Geometry check sheet. Reference: the model listing, model coordinates, mm. A direction names the side the tool comes from. Round coordinates to 2 decimals unless told otherwise and drop trailing zeros. Order: outer loops, then holes, each group sorted by start corner. A loop starts at its lowest first (then second) coordinate and runs counter-clockwise, first axis right, second up.
(1) Draft check along Y on faces 1 (the face through (-18.5, 41, 28)), 2 (the face through (-9.1, 35.83, 27.46)), 3 (the face through (-21.5, 38, 29)). Enter one of: pulls with the +Y half, pulls with the -Y half, needs draft (parallel to the pull), parting line crosses it, or undercut.
(2) Gauge pin test, flat ends, axial feed: P1, Ø5, axis at y = 38, z = 53, coming from the +X side; P2, Ø12.5, axis at x = -23, y = 33, coming from the +Z side; P3, Ø2.5, axis at x = -12.5, z = 27.5, coming from the +Y side. Record the tip position at first contact, or that the pin passes through.
(3) Thickness scan on L1, parallel to Z at x = -97.05, y = 42.65; L2, parallel to X at y = 37.5, z = 35; L3, parallel to X at y = 43.4, z = 17.5. Record the ranges inside material, lowest first.
(4) Set-up check for faces 4 (the face through (-94.1, 40, 38)), 5 (the face through (-31, 28.4, 29)), 6 (the face through (-70, 26, 59)), 7 (the face through (-28, 28, 30)): record each of +Z, -Z, +X, -X, +Y, -Y from which the full face is reachable in a straight line by a thin tool's end or side.
(5) Cross-section at B-B on z = 49. Enter the section's corners in (x, y).
(6) Cross-section at C-C on x = -23. Enter the section's corners in (y, z).
(7) Cross-section at D-D on y = 25. Enter the section's corners in (x, z).
(8) Cross-section at A-A on y = 30.9. Enter the section's corners in (x, z), and give its area (3 significant figures).
from build123d import *

# Parameters (mm, degrees)
SKIZZE1_W                            = 100
SKIZZE1_H                            = 50
AUFSATZ_LINEAR_AUSTRAGEN1_DEPTH      = 10
SERVOLOCH_R                          = 5
SCHNITT_LINEAR_AUSTRAGEN2_DEPTH      = 11
BREITE_W                             = 60
BREITE_H                             = 17
AUFSATZ_LINEAR_AUSTRAGEN2_DEPTH      = 65
SERVO_W                              = 12.1
SERVO_H                              = 23.5
SERVO_R                              = 1.9
SERVO_R_2                            = 1
SCHNITT_LINEAR_AUSTRAGEN3_DEPTH      = 60
F_1_2MM_SCHIENE_W                    = 10
F_1_2MM_SCHIENE_H                    = 65
AUFSATZ_LINEAR_AUSTRAGEN3_DEPTH      = 1.2
SERVOTIEFER_LEGEN_W                  = 12.1
SERVOTIEFER_LEGEN_H                  = 5
SCHNITT_LINEAR_AUSTRAGEN4_DEPTH      = 7.5
F_10_2MM_SCHIENE_W                   = 5.9
F_10_2MM_SCHIENE_H                   = 65
AUFSATZ_LINEAR_AUSTRAGEN4_DEPTH      = 10.2
SCHNITT_LINEAR_AUSTRAGEN5_DEPTH      = 11
SKIZZE11_W                           = 40
SKIZZE11_H                           = 50
SKIZZE11_R                           = 2
AUFSATZ_LINEAR_AUSTRAGEN5_DEPTH      = 20
SKIZZE12_W                           = 40
SKIZZE12_H                           = 50
SCHNITT_LINEAR_AUSTRAGEN6_DEPTH      = 25
SCHNITT_LINEAR_AUSTRAGEN8_DEPTH      = 3
SCHNITT_LINEAR_AUSTRAGEN9_DEPTH      = 46
SCHNITT_LINEAR_AUSTRAGEN9_DEPTH_BACK = 30
VERRUNDUNG5_R                        = 2
VERRUNDUNG6_R                        = 2
VERRUNDUNG7_R                        = 2
SKIZZE14_R                           = 1.25
SCHNITT_LINEAR_AUSTRAGEN10_DEPTH     = 5


with BuildPart() as part:
    # Skizze1 → Aufsatz-Linear austragen1 (new body)
    with BuildSketch(Plane.XY):
        with Locations((-50, 25)):
            Rectangle(SKIZZE1_W, SKIZZE1_H)
    extrude(amount=AUFSATZ_LINEAR_AUSTRAGEN1_DEPTH)

    # ServoLoch → Schnitt-Linear austragen2 (cut, through all)
    with BuildSketch(Plane.XY.offset(10)):
        with Locations((-22.5, 25)):
            Circle(SERVOLOCH_R)
    extrude(amount=-SCHNITT_LINEAR_AUSTRAGEN2_DEPTH, mode=Mode.SUBTRACT)

    # Breite → Aufsatz-Linear austragen2 (add)
    with BuildSketch(Plane.XY.offset(10)):
        with Locations((-70, 25)):
            Rectangle(BREITE_W, BREITE_H)
    extrude(amount=AUFSATZ_LINEAR_AUSTRAGEN2_DEPTH)

    # Servo → Schnitt-Linear austragen3 (cut)
    with BuildSketch(Plane(origin=(0, 33.5, 0), x_dir=(1, 0, 0), z_dir=(0, 1, 0))):
        with Locations((-70, -43.25)):
            Rectangle(SERVO_W, SERVO_H)
        with Locations((-70, -37.5)):
            Circle(SERVO_R, mode=Mode.SUBTRACT)
        with Locations((-70, -37.5)):
            Circle(SERVO_R)
        with Locations((-70, -29)):
            Circle(SERVO_R_2)
        with Locations((-70, -57.5)):
            Circle(SERVO_R_2)
    extrude(amount=-SCHNITT_LINEAR_AUSTRAGEN3_DEPTH, mode=Mode.SUBTRACT)

    # 1,2mm Schiene → Aufsatz-Linear austragen3 (add)
    with BuildSketch(Plane(origin=(0, 33.5, 0), x_dir=(1, 0, 0), z_dir=(0, 1, 0))):
        with Locations((-95, -42.5)):
            Rectangle(F_1_2MM_SCHIENE_W, F_1_2MM_SCHIENE_H)
        with Locations((-45, -42.5)):
            Rectangle(F_1_2MM_SCHIENE_W, F_1_2MM_SCHIENE_H)
    extrude(amount=AUFSATZ_LINEAR_AUSTRAGEN3_DEPTH)

    # ServoTiefer legen → Schnitt-Linear austragen4 (cut)
    with BuildSketch(Plane(origin=(0, 33.5, 0), x_dir=(1, 0, 0), z_dir=(0, 1, 0))):
        with Locations((-70, -29)):
            Rectangle(SERVOTIEFER_LEGEN_W, SERVOTIEFER_LEGEN_H)
        with Locations((-70, -57.5)):
            Rectangle(SERVOTIEFER_LEGEN_W, SERVOTIEFER_LEGEN_H)
    extrude(amount=-SCHNITT_LINEAR_AUSTRAGEN4_DEPTH, mode=Mode.SUBTRACT)

    # 10,2mm Schiene → Aufsatz-Linear austragen4 (add)
    with BuildSketch(Plane(origin=(0, 34.7, 0), x_dir=(1, 0, 0), z_dir=(0, 1, 0))):
        with Locations((-97.05, -42.5)):
            Rectangle(F_10_2MM_SCHIENE_W, F_10_2MM_SCHIENE_H)
        with Locations((-42.95, -42.5)):
            Rectangle(F_10_2MM_SCHIENE_W, F_10_2MM_SCHIENE_H)
    extrude(amount=AUFSATZ_LINEAR_AUSTRAGEN4_DEPTH)

    # Skizze10 → Schnitt-Linear austragen5 (cut, through all)
    with BuildSketch(Plane.XY.offset(10)):
        Polygon((-100, 44.9), (-94.1, 44.9), (-94.1, 34.7), (-90, 34.7), (-90, 33.5), (-50, 33.5), (-50, 34.7), (-45.9, 34.7), (-45.9, 44.9), (-40, 44.9), (-40, 52.602302565), (-100, 52.602302565), align=None)
    extrude(amount=-SCHNITT_LINEAR_AUSTRAGEN5_DEPTH, mode=Mode.SUBTRACT)

    # Skizze11 → Aufsatz-Linear austragen5 (add)
    with BuildSketch(Plane.XY.offset(10)):
        with Locations((-20, 25)):
            Rectangle(SKIZZE11_W, SKIZZE11_H)
        with Locations((-24, 30.9)):
            Circle(SKIZZE11_R, mode=Mode.SUBTRACT)
    extrude(amount=AUFSATZ_LINEAR_AUSTRAGEN5_DEPTH)

    # Skizze12 → Schnitt-Linear austragen6 (cut)
    with BuildSketch(Plane(origin=(0, 0, 0), x_dir=(-1, 0, 0), z_dir=(0, 0, -1))):
        with Locations((20, 25)):
            Rectangle(SKIZZE12_W, SKIZZE12_H)
    extrude(amount=-SCHNITT_LINEAR_AUSTRAGEN6_DEPTH, mode=Mode.SUBTRACT)

    # Skizze15 → Schnitt-Linear austragen8 (cut)
    with BuildSketch(Plane.XY.offset(30)):
        with BuildLine():
            Line((-21.5, 40.9), (-21.5, 34.4))
            ThreePointArc((-21.5, 34.4), (-21.207106781, 33.692893219), (-20.5, 33.4))
            Line((-20.5, 33.4), (-14, 33.4))
            ThreePointArc((-14, 33.4), (-11.5, 30.9), (-14, 28.4))
            Line((-14, 28.4), (-20.5, 28.4))
            ThreePointArc((-20.5, 28.4), (-21.207106781, 28.107106781), (-21.5, 27.4))
            Line((-21.5, 27.4), (-21.5, 20.9))
            ThreePointArc((-21.5, 20.9), (-24, 18.4), (-26.5, 20.9))
            Line((-26.5, 20.9), (-26.5, 27.4))
            ThreePointArc((-26.5, 27.4), (-26.792893219, 28.107106781), (-27.5, 28.4))
            Line((-27.5, 28.4), (-34, 28.4))
            ThreePointArc((-34, 28.4), (-36.5, 30.9), (-34, 33.4))
            Line((-34, 33.4), (-27.5, 33.4))
            ThreePointArc((-27.5, 33.4), (-26.792893219, 33.692893219), (-26.5, 34.4))
            Line((-26.5, 34.4), (-26.5, 40.9))
            ThreePointArc((-26.5, 40.9), (-24, 43.4), (-21.5, 40.9))
        make_face()
    extrude(amount=-SCHNITT_LINEAR_AUSTRAGEN8_DEPTH, mode=Mode.SUBTRACT)

    # Skizze18 → Schnitt-Linear austragen9 (cut, two sides)
    with BuildSketch(Plane.XY.offset(30)) as schnitt_linear_austragen9_sk:
        Polygon((0, 0), (-100, 0), (-100, 16.5), (-8.5, 16.5), (-8.5, 36.4), (-18.5, 36.4), (-18.5, 44.9), (-40, 44.9), (-40, 50), (0, 50), align=None)
    extrude(amount=SCHNITT_LINEAR_AUSTRAGEN9_DEPTH, mode=Mode.SUBTRACT)
    extrude(schnitt_linear_austragen9_sk.sketch, amount=-SCHNITT_LINEAR_AUSTRAGEN9_DEPTH_BACK, mode=Mode.SUBTRACT)

    # Verrundung5
    verrundung5_edges = [part.edges().sort_by_distance(p)[0] for p in [
        (-18.5, 44.9, 27.5),
    ]]
    fillet(verrundung5_edges, radius=VERRUNDUNG5_R)

    # Verrundung6
    verrundung6_edges = [part.edges().sort_by_distance(p)[0] for p in [
        (-18.5, 36.4, 27.5),
    ]]
    fillet(verrundung6_edges, radius=VERRUNDUNG6_R)

    # Verrundung7
    verrundung7_edges = [part.edges().sort_by_distance(p)[0] for p in [
        (-8.5, 36.4, 27.5),
    ]]
    fillet(verrundung7_edges, radius=VERRUNDUNG7_R)

    # Skizze14 → Schnitt-Linear austragen10 (cut)
    with BuildSketch(Plane(origin=(0, 44.9, 0), x_dir=(1, 0, 0), z_dir=(0, 1, 0))):
        with Locations((-97.05, -57.5)):
            Circle(SKIZZE14_R)
        with Locations((-42.95, -57.5)):
            Circle(SKIZZE14_R)
        with Locations((-42.95, -17.5)):
            Circle(SKIZZE14_R)
        with Locations((-97.05, -17.5)):
            Circle(SKIZZE14_R)
    extrude(amount=-SCHNITT_LINEAR_AUSTRAGEN10_DEPTH, mode=Mode.SUBTRACT)


solid = part.part
Found:
1. face 1: needs draft
1. face 2: pulls with the +Y half
1. face 3: undercut
2. P1: stops at x = -40
2. P2: stops at z = 30
2. P3: stops at y = 36.4
3. L1: z = 0 to 16.25, 18.75 to 56.25, 58.75 to 75
3. L2: x = -100 to -94.1, -45.9 to -40
3. L3: x = -100 to -98.3, -95.8 to -94.1, -45.9 to -44.2, -41.7 to -40
4. face 4: +Z, -Z, +Y
4. face 5: +Z
4. face 6: +Y
4. face 7: +Z, +X, +Y, -Y
5. outline: (-100, 16.5) - (-76.05, 16.5) - (-76.05, 33.5) - (-90, 33.5) - (-90, 34.7) - (-94.1, 34.7) - (-94.1, 44.9) - (-100, 44.9) - close; (-63.95, 16.5) - (-40, 16.5) - (-40, 44.9) - (-45.9, 44.9) - (-45.9, 34.7) - (-50, 34.7) - (-50, 33.5) - (-63.95, 33.5) - close
6. outline: (16.5, 25) - (29.17, 25) - (29.17, 27) - (18.61, 27) - (18.61, 30) - (16.5, 30) - close; (32.63, 25) - (44.9, 25) - (44.9, 30) - (43.19, 30) - (43.19, 27) - (32.63, 27) - close
7. outline: (-100, 0) - (-40, 0) - (-40, 25) - (-8.5, 25) - (-8.5, 30) - (-21.5, 30) - (-21.5, 27) - (-26.5, 27) - (-26.5, 30) - (-40, 30) - (-40, 75) - (-100, 75) - close; hole (-76.05, 31.5) - (-63.95, 31.5) - (-63.95, 55) - (-76.05, 55) - close; hole circle Ø2 at (-70, 29); hole circle Ø2 at (-70, 57.5)
8. outline: (-100, 0) - (-40, 0) - (-40, 25) - (-26, 25) - (-26, 27) - (-36.5, 27) - (-36.5, 30) - (-40, 30) - (-40, 75) - (-100, 75) - close; (-22, 25) - (-8.5, 25) - (-8.5, 30) - (-11.5, 30) - (-11.5, 27) - (-22, 27) - close; hole (-76.05, 26.5) - (-63.95, 26.5) - (-63.95, 60) - (-76.05, 60) - close
8. area: 4,170 mm2
